from build123d import *

# Parameters (mm, degrees)
F0_R     = 35
F1_DEPTH = 2
F2_R     = 29.271045
F3_DEPTH = 2
F4_R     = 5
F5_DEPTH = 4


with BuildPart() as f1:
    # F0 (on Top) → F1 (new body)
    with BuildSketch(Plane.XY):
        Circle(F0_R)
    extrude(amount=F1_DEPTH)

    # F2 (on face) → F3 (join)
    with BuildSketch(Plane(origin=(0, 0, 0), x_dir=(1, 0, 0), z_dir=(0, 0, -1))):
        Circle(F2_R)
    extrude(amount=F3_DEPTH)

    # F4 (on face) → F5 (cut, through all)
    with BuildSketch(Plane.XY.offset(2)):
        Circle(F4_R)
    extrude(amount=-F5_DEPTH, mode=Mode.SUBTRACT)


solid = f1.part
Build history of the part. All positions in model axes, mm. A direction names the side the tool comes from. Coordinates: 2 decimals unless noted, no trailing zeros. Order: outer loops, then holes, each group sorted by start corner. A loop starts at its lowest first (then second) coordinate and runs counter-clockwise, first axis right, second up. Notation, with made-up numbers: M 59.25,64 L 72.25,64 A17 cw 72.25,84 Z; hole C 86,53 d4. An arc over 180 degrees is marked long. One line per question, with ' | ' between items. Start each with the question number.
Q1. Saw through at A-A (x = 0). List the corners of the cut face in (y, z), then the cut area to 3 significant figures.
Q2. Probe L1, parallel to Y at x = 0, z = -0.65; L2, parallel to Z at x = 30, y = -14.5; L3, parallel to X at y = 26.5, z = 0.6. List the from-to ranges inside material, lowest first. Write a range as from..to.
Q3. Two-plate mould, pull along Y, no slides. Class faces 3 (the face through (-1.08, -4.88, 0.03)), 4 (the face through (-3.811, -29.022, -0.986)), 5 (the face through (0, 6, -2)): +Y half, -Y half, draft (parallel to the pull), parting line (faces both ways), or undercut.
Q4. Saw through at D-D (x = -7). List the corners of the cut face in (y, z).
Q5. 3-axis set-ups, long thin cutter, end or side, ignore diameter. For faces 1 (the face through (-28, -21, 1)), 2 (the face through (-7.9, -28.4, 0)): which of +Z, -Z, +X, -X, +Y, -Y reach the whole face in a straight line?
Q6. Saw through at C-C (z = 1.4). List the corners of the cut face in (x, y), then the cut area to 3 significant figures.
Q7. Flat gauge pins, fed straight in: pin 1 Ø2 at (x, z) = (2, -1.5) entering from -Y; pin 2 Ø1 at (x, z) = (-26.5, 0) entering from +Y; pin 3 Ø2 at (y, z) = (25, 0.5) entering from +X. Where does each tip first touch, or does it go through?
Check values:
1) outline: M -35,0 L -29.27,0 L -29.27,-2 L -5,-2 L -5,2 L -35,2 Z; M 5,-2 L 29.27,-2 L 29.27,0 L 35,0 L 35,2 L 5,2 Z | area: 217 mm2
2) L1: y = -29.27..-5, 5..29.27 | L2: z = 0..2 | L3: x = -22.86..22.86
3) face 3: undercut | face 4: parting line | face 5: draft
4) outline: M -34.29,0 L -28.42,0 L -28.42,-2 L 28.42,-2 L 28.42,0 L 34.29,0 L 34.29,2 L -34.29,2 Z
5) face 1: +Z, -Z | face 2: -Z
6) outline: C 0,0 d70; hole C 0,0 d10 | area: 3,770 mm2
7) pin 1: stops at y = -29.25 | pin 2: stops at y = 23.43 | pin 3: stops at x = 25.48
